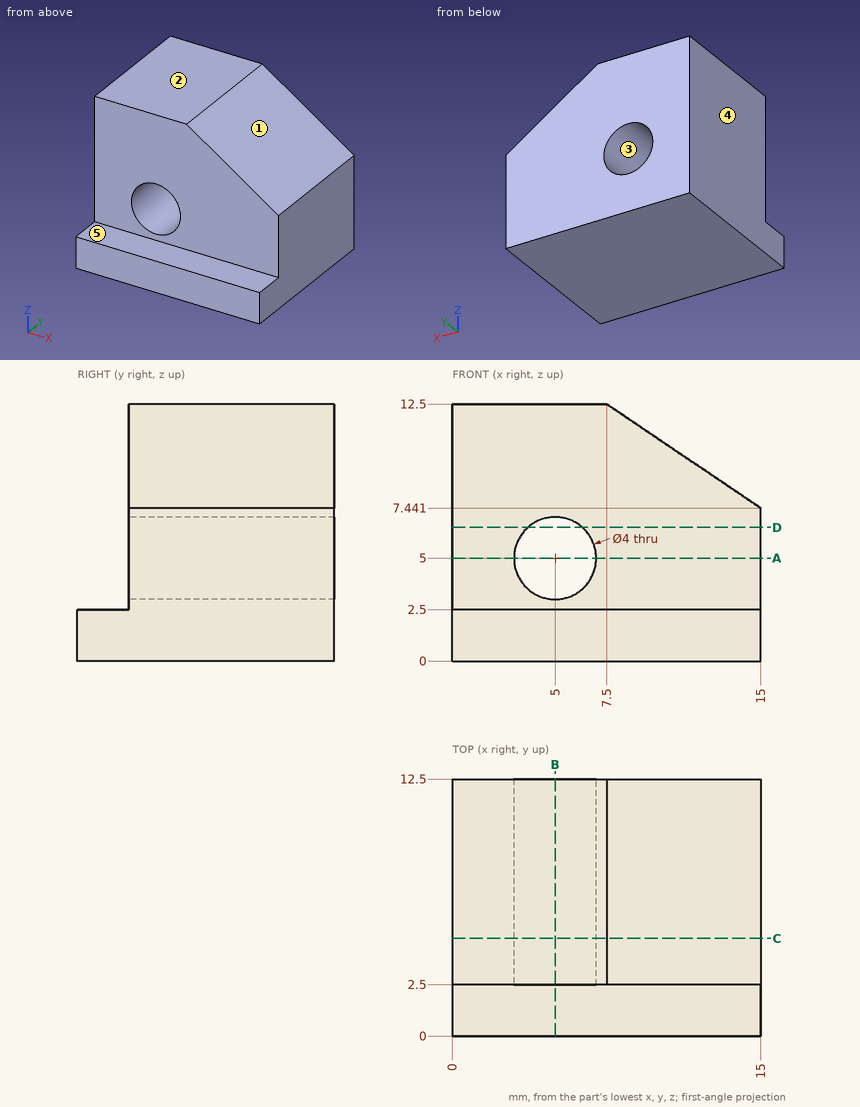
Input: dimensioned drawing with shaded views. Units: mm. Origin: part minimum x, y, z. A direction names the side the tool comes from. Give positions to 0.01 mm unless a question says otherwise; leave off trailing zeros. Order: outer loops, then holes, each group sorted by start corner. A loop starts at its lowest first (then second) coordinate and runs counter-clockwise, first axis right, second up. Notation, with made-up numbers: (69.25, -26.75) -> (106.25, -26.75) arc R33 cw to (106.25, 8.25) -> close; hole circle Ø2 at (-32.5, 50.25). An arc over 180 degrees is marked (long way). Use a Markdown table: item, result.
1) Reachability of the marked faces 4 and 5 from +Z, -Z, +X, -X, +Y, -Y: full face, straight path, thin tool, end or side. Return the list, or none.
Answer list:
| item | result |
|---|---|
| face 4 | +Z, -Z, -X, +Y, -Y |
| face 5 | +Z, +X, -X, -Y |
2) Ray query, line 1 along Z through (x, y) = (5, 4.75); line 2 along Z through (x, y) = (3.25, 9.5); line 3 along Z through (x, y) = (7.25, 2). Return the intervals inside material, ascending. Write a range as [from, to].
Answer list:
| item | result |
|---|---|
| line 1 | [0, 3], [7, 12.5] |
| line 2 | [0, 4.03], [5.97, 12.5] |
| line 3 | [0, 2.5] |
3) Section query A-A, the plane z = 5. Return the cut outline in (x, y), then the cut area to 3 significant figures.
Answer list:
| item | result |
|---|---|
| outline | (0, 2.5) -> (3, 2.5) -> (3, 12.5) -> (0, 12.5) -> close; (7, 2.5) -> (15, 2.5) -> (15, 12.5) -> (7, 12.5) -> close |
| area | 110 mm² |
4) Mould query, pull axis X, two halves, no side actions, for the marked faces 1, 2 and 3. Classes: +X half, -X half, draft (parallel to the pull), parting line (faces both ways), or undercut.
Answer list:
| item | result |
|---|---|
| face 1 | +X half |
| face 2 | draft |
| face 3 | undercut |
5) Contact query for flat-ended pins moving along their axis: P1, Ø5, axis at x = 11.5, y = 10, coming from the +Z side; P2, Ø1, axis at y = 8, z = 9, coming from the +X side; P3, Ø5, axis at x = 5, z = 5.5, coming from the -Y side. Output: stop coordinate, or through.
Answer list:
| item | result |
|---|---|
| P1 | z = 11.49 |
| P2 | x = 13.43 |
| P3 | y = 2.5 |
6) Section query C-C, the plane y = 4.75. Return the cut outline in (x, z), then the cut area to 3 significant figures.
Answer list:
| item | result |
|---|---|
| outline | (0, 0) -> (15, 0) -> (15, 7.44) -> (7.5, 12.5) -> (0, 12.5) -> close; hole circle Ø4 at (5, 5) |
| area | 156 mm² |
7) Section query B-B, the plane x = 5. Return the cut outline in (y, z).
Answer list:
| item | result |
|---|---|
| outline | (0, 0) -> (12.5, 0) -> (12.5, 3) -> (2.5, 3) -> (2.5, 2.5) -> (0, 2.5) -> close; (2.5, 7) -> (12.5, 7) -> (12.5, 12.5) -> (2.5, 12.5) -> close |
8) Section query D-D, the plane z = 6.5. Return the cut outline in (x, y).
Answer list:
| item | result |
|---|---|
| outline | (0, 2.5) -> (3.68, 2.5) -> (3.68, 12.5) -> (0, 12.5) -> close; (6.32, 2.5) -> (15, 2.5) -> (15, 12.5) -> (6.32, 12.5) -> close |
